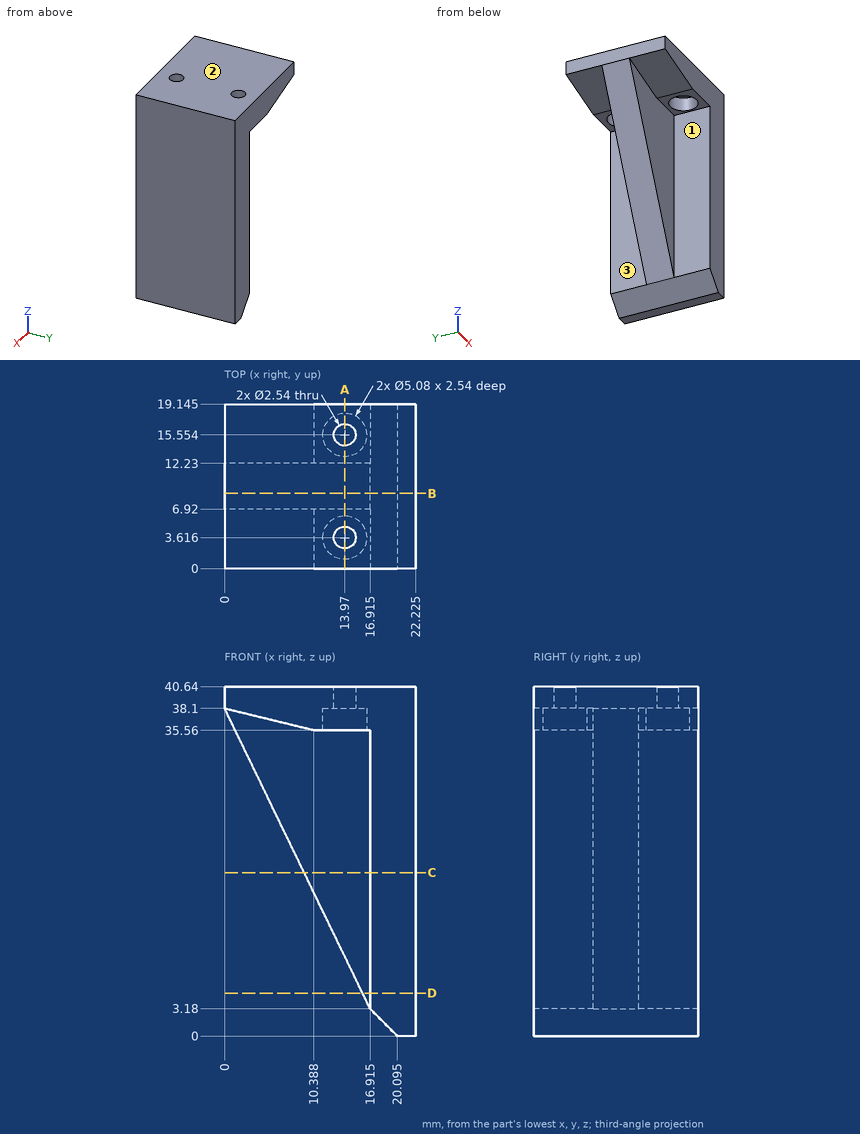
Study the drawing (mm; zero at the part's minimum x, y, z) and answer. A direction names the side the tool comes from. Round coordinates to 2 decimals unless told otherwise and drop trailing zeros. Write each loop counter-clockwise with the first axis right and the second up, starting at its lowest first coordinate (ties: lowest second). Pieces come first, ordered by that corner, then holes. Notation, with made-up numbers: (71, -10.5) - (127, -10.5) arc R25 ccw to (127, 8.5) - close; hole circle Ø2 at (-16.75, -9). An arc over 180 degrees is marked (long way). Return JSON: item names as keys, results as strings. Group by question number.
Q1. The part is cut by section D-D on z = 5. Write down the section's boundary in (x, y) (1 decimal).
Q2. The part is cut by section B-B on y = 8.75. Write down the section's boundary in (x, z) (1 decimal).
Q3. The part is cut by section C-C on z = 19. Write down the section's boundary in (x, y) (1 decimal).
Q4. Each of these flat-tipped pins is pushed along its axis until it touches: pin 1 Ø8 at (y, z) = (9, 33) entering from -X; pin 2 Ø1 at (y, z) = (16.5, 33) entering from -X (3 decimals); pin 3 Ø5 at (x, y) = (14.5, 15) entering from -Z (1 decimal). Where does it stop, or does it pass through?
Q5. Find the intervals of material crossed by L1, parallel to Y at x = 13.97, z = 39.45 (1 decimal); L2, parallel to Y at x = 13.97, z = 36.35 (1 decimal); L3, parallel to X at y = 3, z = 29 (1 decimal), in increasing order.
Q6. The part is cut by section A-A on x = 13.97. Write down the section's boundary in (y, z) (1 decimal), then the cut area to 3 significant figures.
Q7. For the marked faces 1, 2 and 3, determine the directions among +Z, -Z, +X, -X, +Y, -Y from which every point of the face is accessible in a straight line to the end or side of a thin tool.
Solved:
{
 "1": {"outline": "(16, 6.9) - (16.9, 6.9) - (16.9, 0) - (22.2, 0) - (22.2, 19.1) - (16.9, 19.1) - (16.9, 12.2) - (16, 12.2) - close"},
 "2": {"outline": "(0, 38.1) - (16.9, 3.2) - (20.1, 0) - (22.2, 0) - (22.2, 40.6) - (0, 40.6) - close"},
 "3": {"outline": "(9.3, 6.9) - (16.9, 6.9) - (16.9, 0) - (22.2, 0) - (22.2, 19.1) - (16.9, 19.1) - (16.9, 12.2) - (9.3, 12.2) - close"},
 "4": {"pin 1": "x = 0.53", "pin 2": "x = 16.915", "pin 3": "z = 3.1"},
 "5": {"L1": "0 to 2.3, 4.9 to 14.3, 16.8 to 19.1", "L2": "0 to 1.1, 6.2 to 13, 18.1 to 19.1", "L3": "16.9 to 22.2"},
 "6": {"outline": "(0, 35.6) - (1.1, 35.6) - (1.1, 38.1) - (2.3, 38.1) - (2.3, 40.6) - (0, 40.6) - close; (4.9, 38.1) - (6.2, 38.1) - (6.2, 35.6) - (6.9, 35.6) - (6.9, 9.3) - (12.2, 9.3) - (12.2, 35.6) - (13, 35.6) - (13, 38.1) - (14.3, 38.1) - (14.3, 40.6) - (4.9, 40.6) - close; (16.8, 38.1) - (18.1, 38.1) - (18.1, 35.6) - (19.1, 35.6) - (19.1, 40.6) - (16.8, 40.6) - close", "area": "198 mm²"},
 "7": {"face 1": "-Z, -X, -Y", "face 2": "+Z, +X, -X, +Y, -Y", "face 3": "-Z, -X, +Y"}
}
